```python
from build123d import *

# Parameters (mm, degrees)
SKETCH1_R           = 3.5687
BOSS_EXTRUDE1_DEPTH = 19.685
SKETCH2_R           = 2.413
BOSS_EXTRUDE2_DEPTH = 5.715
SKETCH3_R           = 0.2286
BOSS_EXTRUDE3_DEPTH = 3.683
CUT_EXTRUDE1_DEPTH  = 3.683


with BuildPart() as part:
    # Sketch1 → Boss-Extrude1 (new body)
    with BuildSketch(Plane(origin=(0, 0, 0), x_dir=(1, 0, 0), z_dir=(0, 1, 0))):
        with Locations(Location((0, 0, 0), (0, 0, 270))):
            Circle(SKETCH1_R)
    extrude(amount=BOSS_EXTRUDE1_DEPTH)

    # Sketch2 → Boss-Extrude2 (add)
    with BuildSketch(Plane(origin=(0, 19.685, 0), x_dir=(1, 0, 0), z_dir=(0, 1, 0))):
        with Locations(Location((0, 0, 0), (0, 0, 270))):
            Circle(SKETCH2_R)
    extrude(amount=BOSS_EXTRUDE2_DEPTH)

    # Sketch3 → Boss-Extrude3 (add)
    with BuildSketch(Plane.XZ):
        with Locations(Location((1.27, 0, 0), (0, 0, 90))):
            Circle(SKETCH3_R)
        with Locations(Location((-1.27, 0, 0), (0, 0, 90))):
            Circle(SKETCH3_R)
    extrude(amount=BOSS_EXTRUDE3_DEPTH)

    # Sketch4 → Cut-Extrude1 (cut)
    with BuildSketch(Plane.XZ):
        Polygon((2.738767967, 2.287961912), (2.390573782, -2.649674826), (3.144962665, -2.702873114), (4.333390191, 2.287961912), align=None)
    extrude(amount=-CUT_EXTRUDE1_DEPTH, mode=Mode.SUBTRACT)


solid = part.part
```
Build history of the part. All positions in model axes, mm. A direction names the side the tool comes from. Round coordinates to 2 decimals unless told otherwise and drop trailing zeros. Order: outer loops, then holes, each group sorted by start corner. A loop starts at its lowest first (then second) coordinate and runs counter-clockwise, first axis right, second up. Notation, with made-up numbers: (35.5, -19) - (46.5, -19) arc R17 ccw to (46.5, -3) - close; hole circle Ø6 at (29.5, -27). An arc over 180 degrees is marked (long way). Use a Markdown table: item, result.
1) Saw through at A-A on x = 0. Write the cut outline in (y, z) (3 decimals).
Recorded:
| item | result |
|---|---|
| outline | (0, -3.569) - (19.685, -3.569) - (19.685, -2.413) - (25.4, -2.413) - (25.4, 2.413) - (19.685, 2.413) - (19.685, 3.569) - (0, 3.569) - close |
2) Wall check: L1, parallel to Y at x = -2.75, z = 0 (3 decimals); L2, parallel to Y at x = 1, z = 2; L3, parallel to Z at x = -0.5, y = 8.5. Give the ranges that are in metal, low to high.
Recorded:
| item | result |
|---|---|
| L1 | y = 0 to 19.685 |
| L2 | y = 0 to 25.4 |
| L3 | z = -3.53 to 3.53 |
3) Flat gauge pins, fed straight in: pin 1 Ø1.9 at (x, z) = (0, 0) entering from -Y; pin 2 Ø0.6 at (x, z) = (3, -1) entering from -Y; pin 3 Ø3 at (x, y) = (2, 13.5) entering from +Z; pin 4 Ø4 at (x, z) = (2, 2) entering from +Y. Where does each tip first touch, or does it go through?
Recorded:
| item | result |
|---|---|
| pin 1 | stops at y = 0 |
| pin 2 | stops at y = 3.68 |
| pin 3 | stops at z = 3.53 |
| pin 4 | stops at y = 25.4 |
4) Saw through at C-C on z = 0.5. Write the cut outline in (x, y) (1 decimal).
Recorded:
| item | result |
|---|---|
| outline | (-3.5, 0) - (2.6, 0) - (2.6, 3.7) - (3.5, 3.7) - (3.5, 19.7) - (2.4, 19.7) - (2.4, 25.4) - (-2.4, 25.4) - (-2.4, 19.7) - (-3.5, 19.7) - close |
5) Saw through at D-D on z = -1.25. Write the cut outline in (x, y) (3 decimals), and give its area (3 significant figures).
Recorded:
| item | result |
|---|---|
| outline | (-3.343, 0) - (2.489, 0) - (2.489, 3.683) - (3.343, 3.683) - (3.343, 19.685) - (2.064, 19.685) - (2.064, 25.4) - (-2.064, 25.4) - (-2.064, 19.685) - (-3.343, 19.685) - close |
| area | 152 mm² |
6) Tool access for faces 1 (the face through (-1.468, 22.502, -1.915)), 2 (the face through (0, 25.4, 0)), 3 (the face through (2.567, 1.816, -0.146)): list every direction of +Z, -Z, +X, -X, +Y, -Y with a clear straight run to the whole face (end or side of a thin tool).
Recorded:
| item | result |
|---|---|
| face 1 | +Y |
| face 2 | +Z, -Z, +X, -X, +Y |
| face 3 | -Z, +X, -Y |
7) Saw through at B-B on y = 3. Write the cut outline in (x, z).
Recorded:
| item | result |
|---|---|
| outline | (2.39, -2.65) - (2.74, 2.29) arc R3.57 ccw (long way) to start |
